```python
from build123d import *

# Parameters (mm, degrees)
CROQUIS1_R              = 1.6
CROQUIS1_R_2            = 1.4
SALIENTE_EXTRUIR1_DEPTH = 2.5
SALIENTE_EXTRUIR2_START = -32.5
CROQUIS2_R              = 1.4
SALIENTE_EXTRUIR2_DEPTH = 32.5


with BuildPart() as part:
    # Croquis1 → Saliente-Extruir1 (new body)
    with BuildSketch(Plane(origin=(0, 0, 0), x_dir=(1, 0, 0), z_dir=(0, 1, 0))):
        with BuildLine():
            Line((-54.475, -31), (-22.475, -31))
            ThreePointArc((-22.475, -31), (-20.353679656, -30.121320344), (-19.475, -28))
            Line((-19.475, -28), (-19.475, -21.598648019))
            ThreePointArc((-19.475, -21.598648019), (-18.596320344, -19.477327676), (-16.475, -18.598648019))
            Line((-16.475, -18.598648019), (16.135, -18.598648019))
            ThreePointArc((16.135, -18.598648019), (18.256320344, -19.477327676), (19.135, -21.598648019))
            Line((19.135, -21.598648019), (19.135, -28))
            ThreePointArc((19.135, -28), (20.013679656, -30.121320344), (22.135, -31))
            Line((22.135, -31), (51.475, -31))
            ThreePointArc((51.475, -31), (53.596320344, -30.121320344), (54.475, -28))
            Line((54.475, -28), (54.475, -14))
            ThreePointArc((54.475, -14), (53.596320344, -11.878679656), (51.475, -11))
            Line((51.475, -11), (34.52775179, -11))
            ThreePointArc((34.52775179, -11), (32.406431446, -10.121320344), (31.52775179, -8))
            Line((31.52775179, -8), (31.52775179, 8))
            ThreePointArc((31.52775179, 8), (32.406431446, 10.121320344), (34.52775179, 11))
            Line((34.52775179, 11), (51.475, 11))
            ThreePointArc((51.475, 11), (53.596320344, 11.878679656), (54.475, 14))
            Line((54.475, 14), (54.475, 28))
            ThreePointArc((54.475, 28), (53.596320344, 30.121320344), (51.475, 31))
            Line((51.475, 31), (15.953577615, 31))
            ThreePointArc((15.953577615, 31), (13.832257271, 30.121320344), (12.953577615, 28))
            Line((12.953577615, 28), (12.953577615, 22.9600001))
            ThreePointArc((12.953577615, 22.9600001), (12.074897958, 20.838679756), (9.953577615, 19.9600001))
            Line((9.953577615, 19.9600001), (-16.475, 19.9600001))
            ThreePointArc((-16.475, 19.9600001), (-18.596320344, 20.838679756), (-19.475, 22.9600001))
            Line((-19.475, 22.9600001), (-19.475, 28))
            ThreePointArc((-19.475, 28), (-20.353679656, 30.121320344), (-22.475, 31))
            Line((-22.475, 31), (-54.475, 31))
            ThreePointArc((-54.475, 31), (-56.596320344, 30.121320344), (-57.475, 28))
            Line((-57.475, 28), (-57.475, 14))
            ThreePointArc((-57.475, 14), (-56.596320344, 11.878679656), (-54.475, 11))
            Line((-54.475, 11), (-34.52775179, 11))
            ThreePointArc((-34.52775179, 11), (-32.406431446, 10.121320344), (-31.52775179, 8))
            Line((-31.52775179, 8), (-31.52775179, -8))
            ThreePointArc((-31.52775179, -8), (-32.406431446, -10.121320344), (-34.52775179, -11))
            Line((-34.52775179, -11), (-54.475, -11))
            ThreePointArc((-54.475, -11), (-56.596320344, -11.878679656), (-57.475, -14))
            Line((-57.475, -14), (-57.475, -28))
            ThreePointArc((-57.475, -28), (-56.596320344, -30.121320344), (-54.475, -31))
        make_face()
        with Locations(Location((49.495, 25.3400001, 0), (0, 0, 270))):
            Circle(CROQUIS1_R, mode=Mode.SUBTRACT)
        with Locations(Location((-52.075, 26.6, 0), (0, 0, 270))):
            Circle(CROQUIS1_R_2, mode=Mode.SUBTRACT)
        with Locations(Location((-52.075, -26.6, 0), (0, 0, 90))):
            Circle(CROQUIS1_R_2, mode=Mode.SUBTRACT)
        with Locations(Location((-33.04775179, 25.3400001, 0), (0, 0, 270))):
            Circle(CROQUIS1_R, mode=Mode.SUBTRACT)
        with Locations(Location((19.175, 19.9600001, 0), (0, 0, 270))):
            Circle(CROQUIS1_R, mode=Mode.SUBTRACT)
        with Locations(Location((43.175, -23.4799999, 0), (0, 0, 270))):
            Circle(CROQUIS1_R, mode=Mode.SUBTRACT)
        with Locations(Location((-31.52775179, -23.4799999, 0), (0, 0, 270))):
            Circle(CROQUIS1_R, mode=Mode.SUBTRACT)
        with Locations(Location((19.135, -8.1599999, 0), (0, 0, 270))):
            Circle(CROQUIS1_R, mode=Mode.SUBTRACT)
    extrude(amount=SALIENTE_EXTRUIR1_DEPTH)

    # Croquis2 → Saliente-Extruir2 (add)
    # profile 1 of 2: a face of its own
    with BuildSketch(Plane(origin=(0, 2.5, 0), x_dir=(1, 0, 0), z_dir=(0, 1, 0)).offset(SALIENTE_EXTRUIR2_START)):
        Polygon((-55.475, 27.9), (-53.575, 29.8), (-50.575, 29.8), (-48.686440257, 28.294279871), (-48.686440257, 25.304374216), (-50.388696536, 23.00255261), (-53.761303464, 23.00255261), (-55.475, 24.9), align=None)
        with Locations(Location((-52.075, 26.6, 0), (0, 0, 270))):
            Circle(CROQUIS2_R, mode=Mode.SUBTRACT)
    # profile 2 of 2: a face of its own
    with BuildSketch(Plane(origin=(0, 2.5, 0), x_dir=(1, 0, 0), z_dir=(0, 1, 0)).offset(SALIENTE_EXTRUIR2_START)):
        Polygon((-55.475, -27.9), (-53.575, -29.8), (-50.575, -29.8), (-48.686440257, -28.294279871), (-48.686440257, -25.304374216), (-50.388696536, -23.00255261), (-53.761303464, -23.00255261), (-55.475, -24.9), align=None)
        with Locations(Location((-52.075, -26.6, 0), (0, 0, 90))):
            Circle(CROQUIS2_R, mode=Mode.SUBTRACT)
    extrude(amount=SALIENTE_EXTRUIR2_DEPTH)


solid = part.part
```
CAD build for the part. Positions are in the model's coordinates, mm. A direction names the side the tool comes from. Round coordinates to 2 decimals unless told otherwise and drop trailing zeros. Order: outer loops, then holes, each group sorted by start corner. A loop starts at its lowest first (then second) coordinate and runs counter-clockwise, first axis right, second up.
Item 1: Pin check, flat tips, straight feed: pin 1 (0.8 mm diameter, centred on y = 1.5, z = 3.5, fed in from -X); pin 2 (2.5 mm diameter, centred on x = -52.5, y = -7.5, fed in from +Z); pin 3 (2.5 mm diameter, centred on x = -52, y = -13, fed in from -Z). Stop position of each tip, or through.
Item 2: Tool access for faces 1 (the face through (-44, 1, 11)), 2 (the face through (0, 1, 18.599)), 3 (the face through (32.383, 1.232, -10.098)): list every direction of +Z, -Z, +X, -X, +Y, -Y with a clear straight run to the whole face (end or side of a thin tool).
Item 3: Saw through at A-A on y = -17.5. Write the cut outline in (x, z) (3 decimals).
Item 4: Mould opens along Z. For faces 4 (the face through (-20.377, 1.232, 30.145)), 5 (the face through (18.562, 1.232, -18.482)), 6 (the face through (-52, -15, -29.8)) say: pulls with the +Z half, pulls with the -Z half, needs draft (parallel to the pull), parting line crosses it, or undercut.
Item 5: Saw through at B-B on z = 0.5. Write the cut outline in (x, y), then the cut area to 3 significant figures.
Item 6: Probe line 1 along X through (y, z) = (0.8, 23.48) (3 decimals); line 2 along X through (y, z) = (-14, -26.6) (3 decimals); line 3 along X through (y, z) = (1.85, -25.34) (3 decimals). List the from-to ranges inside material, lowest first.
Reported:
1. pin 1: stops at x = -31.53
1. pin 2: stops at z = 29.8
1. pin 3: stops at z = -29.8
2. face 1: -X, +Y, -Y
2. face 2: +Z, +Y, -Y
2. face 3: +X, +Y, -Y
3. outline: (-55.475, -27.9) - (-53.575, -29.8) - (-50.575, -29.8) - (-48.686, -28.294) - (-48.686, -25.304) - (-50.389, -23.003) - (-53.761, -23.003) - (-55.475, -24.9) - close; (-55.475, 24.9) - (-53.761, 23.003) - (-50.389, 23.003) - (-48.686, 25.304) - (-48.686, 28.294) - (-50.575, 29.8) - (-53.575, 29.8) - (-55.475, 27.9) - close; hole circle Ø2.8 at (-52.075, -26.6); hole circle Ø2.8 at (-52.075, 26.6)
4. face 4: pulls with the +Z half
4. face 5: undercut
4. face 6: pulls with the -Z half
5. outline: (-31.53, 0) - (31.53, 0) - (31.53, 2.5) - (-31.53, 2.5) - close
5. area: 158 mm2
6. line 1: x = -57.475 to -33.128, -29.928 to -19.475, 19.135 to 41.575, 44.775 to 54.475
6. line 2: x = -55.475 to -53.475, -50.675 to -48.686
6. line 3: x = -57.475 to -52.685, -51.465 to -34.648, -31.448 to -19.475, 12.954 to 47.895, 51.095 to 54.475
